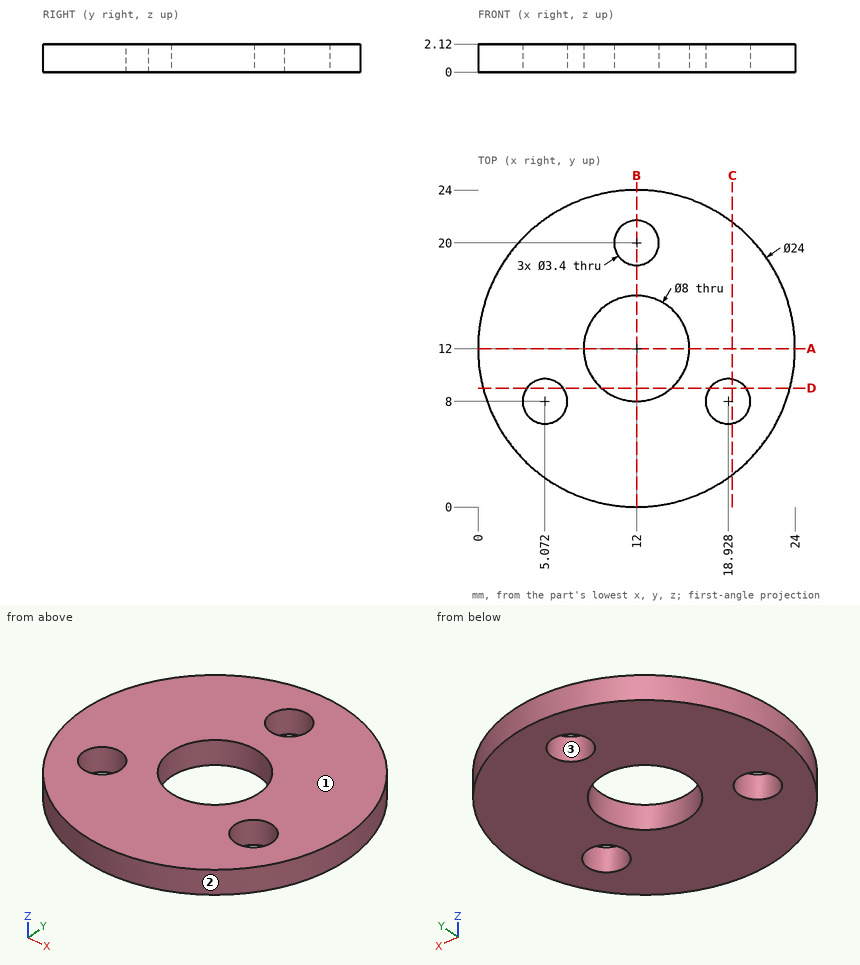
Answer from the drawing. Dimensions are ordinates in mm from the lowest x, y and z of the part. Coordinates: 2 decimals unless noted, no trailing zeros. Order: outer loops, then holes, each group sorted by start corner. A loop starts at its lowest first (then second) coordinate and runs counter-clockwise, first axis right, second up. Notation, with made-up numbers: (-9.5, 21.25) - (42.5, 21.25) arc R34 ccw to (42.5, 54.25) - close; hole circle Ø1 at (34.5, 22.5). An arc over 180 degrees is marked (long way). Put each result on its own line as item: value. Start each with the question number.
1) Find the intervals of material crossed by line 1 (Y direction, x = 10.5, z = 0.1) (1 decimal); line 2 (Y direction, x = 19, z = 1.6); line 3 (X direction, y = 20, z = 0.75) (1 decimal), in increasing order. Write a range as from..to.
2) Flat-ended cylindrical pins translate along their axes: pin 1 (1 mm diameter, centred on x = 10.5, z = 1, fed in from +Y); pin 2 (1 mm diameter, centred on x = 16.5, z = 2, fed in from -Y). Find the tip coordinate at first contact, or state that the pin passes through.
3) Find section B-B (x = 12). Give the vertices of the cut face in (y, z).
4) Find section D-D (y = 9). Give the vertices of the cut face in (x, z).
5) Find section A-A (y = 12). Give the vertices of the cut face in (x, z), plus the area to 3 significant figures.
6) Find section C-C (x = 19.25). Give the vertices of the cut face in (y, z).
7) For a pull along Y with two mould halves and no side action, classify the marked faces 1, 2 and 3 as released by +Y, released by -Y, zero draft, split by the parting line, or undercut.
Results list:
1. line 1: y = 0.1..8.3, 15.7..19.2, 20.8..23.9
1. line 2: y = 2.25..6.3, 9.7..21.75
1. line 3: x = 3.1..10.3, 13.7..20.9
2. pin 1: stops at y = 23.96
2. pin 2: stops at y = 0.69
3. outline: (0, 0) - (8, 0) - (8, 2.12) - (0, 2.12) - close; (16, 0) - (18.3, 0) - (18.3, 2.12) - (16, 2.12) - close; (21.7, 0) - (24, 0) - (24, 2.12) - (21.7, 2.12) - close
4. outline: (0.38, 0) - (3.7, 0) - (3.7, 2.12) - (0.38, 2.12) - close; (6.45, 0) - (9.35, 0) - (9.35, 2.12) - (6.45, 2.12) - close; (14.65, 0) - (17.55, 0) - (17.55, 2.12) - (14.65, 2.12) - close; (20.3, 0) - (23.62, 0) - (23.62, 2.12) - (20.3, 2.12) - close
5. outline: (0, 0) - (8, 0) - (8, 2.12) - (0, 2.12) - close; (16, 0) - (24, 0) - (24, 2.12) - (16, 2.12) - close
5. area: 33.9 mm^2
6. outline: (2.44, 0) - (6.33, 0) - (6.33, 2.12) - (2.44, 2.12) - close; (9.67, 0) - (21.56, 0) - (21.56, 2.12) - (9.67, 2.12) - close
7. face 1: zero draft
7. face 2: split by the parting line
7. face 3: undercut
